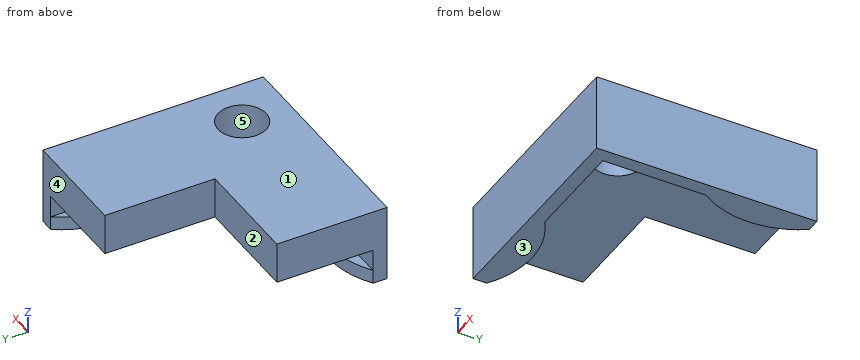
from build123d import *

# Parameters (mm, degrees)
ESQUISSE1_R        = 1.75
BOSS_EXTRU_1_DEPTH = 3
BOSS_EXTRU_2_DEPTH = 5.6
BOSS_EXTRU_3_DEPTH = 1


with BuildPart() as part:
    # Esquisse1 → Boss.-Extru.1 (new body)
    with BuildSketch(Plane.XY):
        Polygon((104.864902494, -135.367060458), (89.864902494, -135.367060458), (89.864902494, -128.367060458), (97.864902494, -128.367060458), (97.864902494, -120.367060458), (104.864902494, -120.367060458), align=None)
        with Locations((102.364902494, -132.867060458)):
            Circle(ESQUISSE1_R, mode=Mode.SUBTRACT)
    extrude(amount=BOSS_EXTRU_1_DEPTH)

    # Esquisse2 → Boss.-Extru.2 (add)
    with BuildSketch(Plane.XY.offset(3)):
        Polygon((89.864902494, -135.367060458), (89.864902494, -136.367060458), (105.864902494, -136.367060458), (105.864902494, -120.367060458), (104.864902494, -120.367060458), (104.864902494, -135.367060458), align=None)
    extrude(amount=-BOSS_EXTRU_2_DEPTH)

    # Esquisse3 → Boss.-Extru.3 (add)
    with BuildSketch(Plane(origin=(0, 0, -2.6), x_dir=(-1, 0, 0), z_dir=(0, 0, -1))):
        with BuildLine():
            Line((-89.864902494, -135.367060458), (-97.364902494, -135.367060458))
            ThreePointArc((-97.364902494, -135.367060458), (-93.614902494, -134.19740032), (-89.864902494, -135.367060458))
        make_face()
        with BuildLine():
            Line((-104.864902494, -127.867060458), (-104.864902494, -120.367060458))
            ThreePointArc((-104.864902494, -120.367060458), (-103.695242356, -124.117060458), (-104.864902494, -127.867060458))
        make_face()
    extrude(amount=-BOSS_EXTRU_3_DEPTH)


solid = part.part
Geometry: final body of the model. Coordinates: model frame, mm. Face numbers are marked on the shaded views. A direction names the side the tool comes from. Round coordinates to 2 decimals unless told otherwise and drop trailing zeros. Loops run counter-clockwise (first coordinate to the right, second up) from the corner with the lowest first, then second, coordinate; pieces in that order, holes last. Notation, with made-up numbers: M 44,54 L 97,54 A17 ccw 97,83 Z; hole C 60,10 d4. An arc over 180 degrees is marked long. Put each result on its own line as item: value. Start each with the question number.
(1) Section query A-A (y = -131.75). Return loops of the section in (x, z).
(2) Contact query for flat-ended pins moving along their axis: pin 1 Ø1.3 at (y, z) = (-130, -1) entering from -X; pin 2 Ø4 at (x, y) = (100, -128) entering from -Z; pin 3 Ø4 at (x, y) = (102.36, -132.87) entering from +Z; pin 4 Ø0.9 at (x, z) = (93, 1.5) entering from +Y. Output: stop coordinate, or through.
(3) Set-up query: the marked faces 1 and 2. Return all of +Z, -Z, +X, -X, +Y, -Y with unobstructed straight access to the full face (end or side cutting, diameter ignored); none if empty.
(4) Draft query along Y for the marked faces 3, 4 and 5. Return one class per face: +Y half, -Y half, draft (parallel to the pull), parting line (faces both ways), or undercut.
(5) Section query B-B (z = -1.9). Return loops of the section in (x, y).
(6) Material intervals for line 1 along X through (y, z) = (-133, 1.1); line 2 along Z through (x, y) = (91.5, -129.25); line 3 along Y through (x, z) = (93.5, -0.75), sorted ascending. Write a range as [from, to].
(7) Section query D-D (z = 2.25). Return loops of the section in (x, y), then the cut area to 3 significant figures.
(8) Section query C-C (x = 102). Return loops of the section in (y, z), then the cut area to 3 significant figures.
Findings below:
1. outline: M 89.86,0 L 101.02,0 L 101.02,3 L 89.86,3 Z; M 103.71,0 L 104.86,0 L 104.86,-2.6 L 105.86,-2.6 L 105.86,3 L 103.71,3 Z
2. pin 1: stops at x = 104.86
2. pin 2: stops at z = 0
2. pin 3: stops at z = 3
2. pin 4: stops at y = -128.37
3. face 1: +Z, +X, -X, +Y, -Y
3. face 2: +Z, -Z, -X, +Y
4. face 3: draft
4. face 4: +Y half
4. face 5: undercut
5. outline: M 89.86,-136.37 L 105.86,-136.37 L 105.86,-120.37 L 104.86,-120.37 A6.6 ccw 104.86,-127.87 L 104.86,-135.37 L 97.36,-135.37 A6.6 ccw 89.86,-135.37 Z
6. line 1: x = [89.86, 100.62], [104.11, 105.86]
6. line 2: z = [0, 3]
6. line 3: y = [-136.37, -135.37]
7. outline: M 89.86,-136.37 L 105.86,-136.37 L 105.86,-120.37 L 97.86,-120.37 L 97.86,-128.37 L 89.86,-128.37 Z; hole C 102.36,-132.87 d3.5
7. area: 182 mm2
8. outline: M -136.37,-2.6 L -135.37,-2.6 L -135.37,0 L -134.58,0 L -134.58,3 L -136.37,3 Z; M -131.16,0 L -120.37,0 L -120.37,3 L -131.16,3 Z
8. area: 40.3 mm2
